```python
from build123d import *

# Parameters (mm, degrees)
F1_DEPTH = 6.35
F2_DEPTH = 38.1
F3_R     = 6.34999


# Not quite as in the source:
# - a fillet or chamfer is up to 0.001 mm smaller than in the source, because OpenCascade refuses the exact size


with BuildPart() as f1:
    # F0 (on Top) → F1 (new body)
    with BuildSketch(Plane.XY):
        with BuildLine():
            Line((-19.05, -38.1000031829), (19.05, -38.1000031829))
            ThreePointArc((19.05, -38.1000031829), (32.5203864322, -32.5203864322), (38.1000031829, -19.05))
            Line((38.1000031829, -19.05), (38.1000031829, 19.05))
            ThreePointArc((38.1000031829, 19.05), (32.5203864322, 32.5203864322), (19.05, 38.1000031829))
            Line((19.05, 38.1000031829), (-19.05, 38.1000031829))
            ThreePointArc((-19.05, 38.1000031829), (-32.5203864322, 32.5203864322), (-38.1000031829, 19.05))
            Line((-38.1000031829, 19.05), (-38.1000031829, -19.05))
            ThreePointArc((-38.1000031829, -19.05), (-32.5203864322, -32.5203864322), (-19.05, -38.1000031829))
        make_face()
        with BuildLine():
            ThreePointArc((-19.05, -31.75), (-28.0302561211, -28.0302561211), (-31.75, -19.05))
            Line((-31.75, -19.05), (-31.75, 19.05))
            ThreePointArc((-31.75, 19.05), (-28.0302561211, 28.0302561211), (-19.05, 31.75))
            Line((-19.05, 31.75), (19.05, 31.75))
            ThreePointArc((19.05, 31.75), (28.0302561211, 28.0302561211), (31.75, 19.05))
            Line((31.75, 19.05), (31.75, -19.05))
            ThreePointArc((31.75, -19.05), (28.0302561211, -28.0302561211), (19.05, -31.75))
            Line((19.05, -31.75), (-19.05, -31.75))
        make_face(mode=Mode.SUBTRACT)
        with BuildLine():
            Line((-31.75, 19.05), (-31.75, -19.05))
            ThreePointArc((-31.75, -19.05), (-28.0302561211, -28.0302561211), (-19.05, -31.75))
            Line((-19.05, -31.75), (19.05, -31.75))
            ThreePointArc((19.05, -31.75), (28.0302561211, -28.0302561211), (31.75, -19.05))
            Line((31.75, -19.05), (31.75, 19.05))
            ThreePointArc((31.75, 19.05), (28.0302561211, 28.0302561211), (19.05, 31.75))
            Line((19.05, 31.75), (-19.05, 31.75))
            ThreePointArc((-19.05, 31.75), (-28.0302561211, 28.0302561211), (-31.75, 19.05))
        make_face()
        with BuildLine():
            Line((19.05, -25.4), (-19.05, -25.4))
            ThreePointArc((-19.05, -25.4), (-23.5401280605, -23.5401280605), (-25.4, -19.05))
            Line((-25.4, -19.05), (-25.4, 19.05))
            ThreePointArc((-25.4, 19.05), (-23.5401280605, 23.5401280605), (-19.05, 25.4))
            Line((-19.05, 25.4), (19.05, 25.4))
            ThreePointArc((19.05, 25.4), (23.5401280605, 23.5401280605), (25.4, 19.05))
            Line((25.4, 19.05), (25.4, -19.05))
            ThreePointArc((25.4, -19.05), (23.5401280605, -23.5401280605), (19.05, -25.4))
        make_face(mode=Mode.SUBTRACT)
    extrude(amount=F1_DEPTH)

    # F0 (on Top) → F2 (join)
    with BuildSketch(Plane.XY):
        with BuildLine():
            Line((-31.75, 19.05), (-31.75, -19.05))
            ThreePointArc((-31.75, -19.05), (-28.0302561211, -28.0302561211), (-19.05, -31.75))
            Line((-19.05, -31.75), (19.05, -31.75))
            ThreePointArc((19.05, -31.75), (28.0302561211, -28.0302561211), (31.75, -19.05))
            Line((31.75, -19.05), (31.75, 19.05))
            ThreePointArc((31.75, 19.05), (28.0302561211, 28.0302561211), (19.05, 31.75))
            Line((19.05, 31.75), (-19.05, 31.75))
            ThreePointArc((-19.05, 31.75), (-28.0302561211, 28.0302561211), (-31.75, 19.05))
        make_face()
        with BuildLine():
            Line((19.05, -25.4), (-19.05, -25.4))
            ThreePointArc((-19.05, -25.4), (-23.5401280605, -23.5401280605), (-25.4, -19.05))
            Line((-25.4, -19.05), (-25.4, 19.05))
            ThreePointArc((-25.4, 19.05), (-23.5401280605, 23.5401280605), (-19.05, 25.4))
            Line((-19.05, 25.4), (19.05, 25.4))
            ThreePointArc((19.05, 25.4), (23.5401280605, 23.5401280605), (25.4, 19.05))
            Line((25.4, 19.05), (25.4, -19.05))
            ThreePointArc((25.4, -19.05), (23.5401280605, -23.5401280605), (19.05, -25.4))
        make_face(mode=Mode.SUBTRACT)
    extrude(amount=-F2_DEPTH)

    # F3 (radius 6.35 in the source; OpenCascade refuses exactly that, so slightly less here)
    f3_edges = [f1.edges().sort_by_distance(p)[0] for p in [
        (23.540128, -23.540128, 6.35),
        (0, -25.4, 6.35),
        (-23.540128, -23.540128, 6.35),
        (-25.4, 0, 6.35),
        (-23.540128, 23.540128, 6.35),
        (0, 25.4, 6.35),
        (23.540128, 23.540128, 6.35),
        (25.4, 0, 6.35),
        (0, -38.100003, 6.35),
        (32.520386, -32.520386, 6.35),
        (38.100003, 0, 6.35),
        (32.520386, 32.520386, 6.35),
        (0, 38.100003, 6.35),
        (-32.520386, 32.520386, 6.35),
        (-38.100003, 0, 6.35),
        (-32.520386, -32.520386, 6.35),
    ]]
    fillet(f3_edges, radius=F3_R)


solid = f1.part
```
The listing builds one solid part. Answer for the finished solid, in the listing's coordinates (mm). A direction names the side the tool comes from. Give positions to 0.01 mm unless a question says otherwise; leave off trailing zeros. Write each loop counter-clockwise with the first axis right and the second up, starting at its lowest first coordinate (ties: lowest second). Pieces come first, ordered by that corner, then holes. Notation, with made-up numbers: M 30.5,26 L 86.5,26 A19 cw 86.5,58 Z; hole C 89,-20.5 d5. An arc over 180 degrees is marked long. Write each question's results on one line, items separated by ' | '.
Q1. Consider L1, parallel to X at y = -8, z = -7.5; L2, parallel to X at y = -3.5, z = 0.5. Determine where each line is inside the solid, lowest interval first. Write a range as from..to.
Output values:
L1: -31.75..-25.4, 25.4..31.75 | L2: -38.08..-25.42, 25.42..38.08
Q2. Section C-C, the plane z = -21 is taken. Write down the section's boundary in (x, y).
Output values:
outline: M -31.75,-19.05 A12.7 ccw -19.05,-31.75 L 19.05,-31.75 A12.7 ccw 31.75,-19.05 L 31.75,19.05 A12.7 ccw 19.05,31.75 L -19.05,31.75 A12.7 ccw -31.75,19.05 Z; hole M -25.4,-19.05 A6.35 ccw -19.05,-25.4 L 19.05,-25.4 A6.35 ccw 25.4,-19.05 L 25.4,19.05 A6.35 ccw 19.05,25.4 L -19.05,25.4 A6.35 ccw -25.4,19.05 Z
Q3. Section D-D, the plane z = 3.5 is taken. Write down the section's boundary in (x, y), then the cut area to 3 significant figures.
Output values:
outline: M -37.05,-19.05 A18 ccw -19.05,-37.05 L 19.05,-37.05 A18 ccw 37.05,-19.05 L 37.05,19.05 A18 ccw 19.05,37.05 L -19.05,37.05 A18 ccw -37.05,19.05 Z; hole M -26.45,-19.05 A7.4 ccw -19.05,-26.45 L 19.05,-26.45 A7.4 ccw 26.45,-19.05 L 26.45,19.05 A7.4 ccw 19.05,26.45 L -19.05,26.45 A7.4 ccw -26.45,19.05 Z | area: 2,460 mm2
Q4. For a pull along Y with two mould halves and no side action, classify faces 1 (the cylindrical face through (28.13, 27.93, -18.78)), 2 (the flat face through (25.4, 0, -19)), 3 (the cylindrical face through (-28.13, -27.93, -18.78)), 4 (the flat face through (31.75, 0, -19)) as released by +Y, released by -Y, zero draft, split by the parting line, or undercut.
Output values:
face 1: released by +Y | face 2: undercut | face 3: released by -Y | face 4: zero draft
Q5. Flat-ended cylindrical pins translate along their axes: P1, Ø19, axis at x = 8, z = -27, coming from the -Y side; P2, Ø10, axis at x = -22.5, z = -15.5, coming from the +Y side; P3, Ø5, axis at y = 10.5, z = -9, coming from the +X side. Find the tip coordinate at first contact, or state that the pin passes through.
Output values:
P1: y = -31.75 | P2: y = 31.75 | P3: x = 31.75
Q6. A tool of negligible diameter and unlimited length cuts with its end or side. For faces 5 (the flat face through (0, -31.75, -19)), 6 (the flat face through (0, 25.4, -19)), 7 (the cylindrical face through (-0.27, -27.31, 4.54)), from which of +Z, -Z, +X, -X, +Y, -Y can it reach the whole face along a straight path? Write none if from no direction.
Output values:
face 5: -Z, +X, -X, -Y | face 6: +Z, -Z | face 7: +Z
